```python
from build123d import *

# Parameters (mm, degrees)
SKETCH1_W           = 24.13
SKETCH1_H           = 31.75
BOSS_EXTRUDE1_DEPTH = 2.54
BOSS_EXTRUDE2_DEPTH = 2.54
SKETCH3_W           = 31.75
SKETCH3_H           = 5.08
CUT_EXTRUDE1_DEPTH  = 2.54
BOSS_EXTRUDE3_DEPTH = 2.54
SKETCH5_R           = 2.5527
BOSS_EXTRUDE4_DEPTH = 2.54


with BuildPart() as part:
    # Sketch1 → Boss-Extrude1 (new body)
    with BuildSketch(Plane(origin=(0, 0, 0), x_dir=(1, 0, 0), z_dir=(0, 1, 0))):
        Rectangle(SKETCH1_W, SKETCH1_H)
    extrude(amount=BOSS_EXTRUDE1_DEPTH)

    # Sketch2 → Boss-Extrude2 (add)
    with BuildSketch(Plane(origin=(0, 2.54, 0), x_dir=(1, 0, 0), z_dir=(0, 1, 0))):
        Polygon((-12.065, 15.875), (-12.065, 13.335), (-9.525, 13.335), (9.525, 13.335), (9.525, -13.335), (-9.525, -13.335), (-12.065, -13.335), (-12.065, -15.875), (12.065, -15.875), (12.065, 15.875), align=None)
    extrude(amount=BOSS_EXTRUDE2_DEPTH)

    # Sketch3 → Cut-Extrude1 (cut)
    with BuildSketch(Plane.ZY.offset(12.065)):
        with Locations((0, 2.54)):
            Rectangle(SKETCH3_W, SKETCH3_H)
    extrude(amount=-CUT_EXTRUDE1_DEPTH, mode=Mode.SUBTRACT)

    # Sketch4 → Boss-Extrude3 (add)
    with BuildSketch(Plane(origin=(0, 5.08, 0), x_dir=(1, 0, 0), z_dir=(0, 1, 0))):
        Polygon((-9.525, 15.875), (-9.525, 12.7), (8.509, 12.7), (8.509, -11.43), (-9.525, -11.43), (-9.525, -15.875), (12.065, -15.875), (12.065, 15.875), align=None)
    extrude(amount=BOSS_EXTRUDE3_DEPTH)

    # Sketch5 → Boss-Extrude4 (add)
    # profile 1 of 2: a face of its own
    with BuildSketch(Plane(origin=(0, 0, 0), x_dir=(-1, 0, 0), z_dir=(0, -1, 0))):
        with BuildLine():
            Line((-12.065, 6.35), (-12.065, -6.35))
            Line((-12.065, -6.35), (-18.415, -6.35))
            ThreePointArc((-18.415, -6.35), (-22.905128061, -4.490128061), (-24.765, 0))
            ThreePointArc((-24.765, 0), (-22.905128061, 4.490128061), (-18.415, 6.35))
            Line((-18.415, 6.35), (-12.065, 6.35))
        make_face()
        with Locations((-18.415, 0)):
            Circle(SKETCH5_R, mode=Mode.SUBTRACT)
    # profile 2 of 2: a face of its own
    with BuildSketch(Plane(origin=(0, 0, 0), x_dir=(-1, 0, 0), z_dir=(0, -1, 0))):
        with BuildLine():
            Line((9.525, 6.35), (15.875, 6.35))
            ThreePointArc((15.875, 6.35), (20.365128061, 4.490128061), (22.225, 0))
            ThreePointArc((22.225, 0), (20.365128061, -4.490128061), (15.875, -6.35))
            Line((15.875, -6.35), (9.525, -6.35))
            Line((9.525, -6.35), (9.525, 6.35))
        make_face()
        with Locations((15.875, 0)):
            Circle(SKETCH5_R, mode=Mode.SUBTRACT)
    extrude(amount=BOSS_EXTRUDE4_DEPTH)


with BuildPart() as boss_extrude4_kept_piece:
    # of the separate pieces the step leaves, the one the design keeps (boss_extrude4_pieces_kept)
    add(part.part.solids().sort_by_distance((12.065, 0, 15.875))[0])


solid = boss_extrude4_kept_piece.part
```
Source: CAD feature listing. Evaluate the final solid. Frame: model axes, mm. A direction names the side the tool comes from. Coordinates: 2 decimals unless noted, no trailing zeros. Write each loop counter-clockwise with the first axis right and the second up, starting at its lowest first coordinate (ties: lowest second). Pieces come first, ordered by that corner, then holes. Notation, with made-up numbers: M -9,-20.75 L 6,-20.75 A26 cw 6,4.25 Z; hole C 26,43.25 d11. An arc over 180 degrees is marked long. Answer as a JSON object with one key per item and string values.
1. Cut plane B-B on z = 6. Output: boundary loops of the cut face in (x, y) (3 decimals), plus the area to 3 significant figures.
Evaluation:
{"outline": "M -9.525,0 L 12.065,0 L 12.065,7.62 L 8.509,7.62 L 8.509,5.08 L 9.525,5.08 L 9.525,2.54 L -9.525,2.54 Z", "area": "70.3 mm^2"}
2. Access query for faces 1 (the flat face through (12.065, 4, 0)), 2 (the flat face through (-1, 6, -12.7)), 3 (the flat face through (0, 4, 13.335)). Directions: +Z, -Z, +X, -X, +Y, -Y. A direction counts if a zero-diameter tool reaches every point of the face in a straight line with its end or side. Return the directions, or none.
Evaluation:
{"face 1": "+Z, -Z, +X, +Y, -Y", "face 2": "-X, +Y", "face 3": "-X"}
3. Ray query, L1, parallel to Z at x = -2, y = 5.5 (3 decimals); L2, parallel to Z at x = -3.25, y = 5 (3 decimals); L3, parallel to X at y = 6, z = -5 (3 decimals). Return the intervals inside material, ascending.
Evaluation:
{"L1": "-15.875 to -12.7, 11.43 to 15.875", "L2": "-15.875 to -13.335, 13.335 to 15.875", "L3": "8.509 to 12.065"}
4. Cut plane A-A on y = 3.5. Output: boundary loops of the cut face in (x, z) (3 decimals).
Evaluation:
{"outline": "M -9.525,-15.875 L 12.065,-15.875 L 12.065,15.875 L -9.525,15.875 L -9.525,13.335 L 9.525,13.335 L 9.525,-13.335 L -9.525,-13.335 Z"}
5. Contact query for flat-ended pins moving along their axis: P1, Ø2, axis at x = 4.5, z = -5, coming from the +Y side; P2, Ø3, axis at y = 6.5, z = 3.5, coming from the -X side; P3, Ø0.8, axis at y = 3.5, z = 3.5, coming from the -X side (3 decimals). Output: stop coordinate, or through.
Evaluation:
{"P1": "y = 2.54", "P2": "x = 8.51", "P3": "x = 9.525"}
6. Cut plane C-C on x = 0. Output: boundary loops of the cut face in (y, z) (3 decimals), plus the area to 3 significant figures.
Evaluation:
{"outline": "M 0,-15.875 L 7.62,-15.875 L 7.62,-12.7 L 5.08,-12.7 L 5.08,-13.335 L 2.54,-13.335 L 2.54,13.335 L 5.08,13.335 L 5.08,11.43 L 7.62,11.43 L 7.62,15.875 L 0,15.875 Z", "area": "113 mm^2"}
7. Draft query along Z for faces 4 (the flat face through (0, 2.54, 0)), 5 (the flat face through (-9.525, 2, 0)), 6 (the flat face through (1, 4, 15.875)), 7 (the flat face through (1, 4, -15.875)). Return one class per face: released by +Z, released by -Z, zero draft, split by the parting line, or undercut.
Evaluation:
{"face 4": "undercut", "face 5": "zero draft", "face 6": "released by +Z", "face 7": "released by -Z"}
